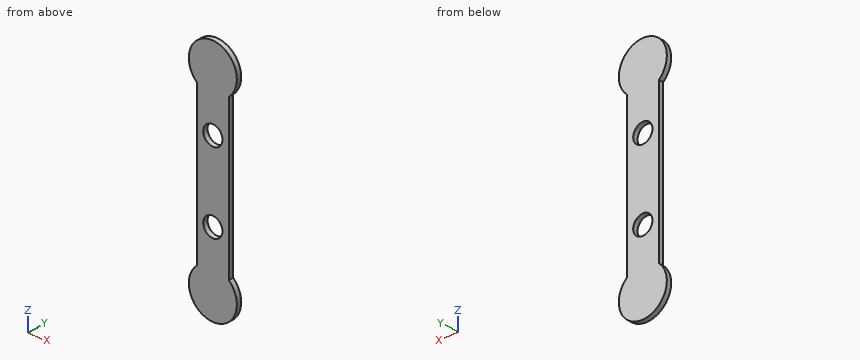
Autodesk Inventor part; units mm, degrees
ref_plane "YZ Plane" through (0, 0, 0) normal (1, 0, 0) x (0, 1, 0)
ref_plane "XZ Plane" through (0, 0, 0) normal (0, 1, 0) x (-1, 0, 0)
ref_plane "XY Plane" through (0, 0, 0) normal (0, 0, 1) x (1, 0, 0)
sketch "Sketch1" plane through (0, 0, 0) normal (0, 1, 0) x (-1, 0, 0)
  line L0 (0, 0) -> (0, 75)
  line L1 (0, 0) -> (0, -75)
  line L2 (0, -75) -> (0, -60)
  circle A0 centre (0, -60) radius 15
  circle A1 centre (0, 60) radius 15
  line L3 (-10, 45) -> (-10, -48.8197)
  line L4 (10, 45) -> (10, -48.8197)
  line L5 (10, 45) -> (10, 48.8197)
  line L6 (-10, 45) -> (-10, 48.8197)
  line L7 (10, 45) -> (-10, 45)
  line L8 (-10, -48.8197) -> (-10, 0)
  line L9 (0, -24.4098) -> (10, -24.4098)
  line L10 (10, 0) -> (0, 0)
  line L11 (0, 24.4098) -> (10, 24.4098)
  line L12 (0, -24.4098) -> (-10, -24.4098)
  line L13 (0, 24.4098) -> (-10, 24.4098)
  circle A2 centre (0, -24.4098) radius 6
  circle A3 centre (0, 24.4098) radius 6
  dimension "d1" = 75
  dimension "d2" = 75
  dimension "d3" = 15
  dimension "d6" = 20
  dimension "d7" = 97.6393
  dimension "d10" = 12
  dimension "d11" = 12
extrude "Extrusion1" add sketch "Sketch1" along normal blind 3 contours L1 A2 L12 L3 L13 A3 L0 | L10 L4 L9 A2 L1 | L0 A3 L11 L4 L10 | L13 L3 L7 L0 A3 | A3 L0 L7 L4 L11 | L9 L4 A0 L1 A2 | A2 L1 A0 L3 L12 | L7 A1 L5 | A0 L1 | A1 L0 | L7 L6 A1 | L0 A1 | L1 A0
properties part number "ramenovaPricka"
Input: part model. Units: mm. Frame: model coordinates. Coordinates: 2 decimals unless noted, no trailing zeros. Loops run counter-clockwise (first coordinate to the right, second up) from the corner with the lowest first, then second, coordinate; pieces in that order, holes last. Notation, with made-up numbers: (-37.75, -21) -> (-15.75, -21) arc R36 cw to (-15.75, 17) -> close; hole circle Ø11 at (89.25, -6). An arc over 180 degrees is marked (long way). Write each question's results on one line, items separated by ' | '. Start each with the question number.
Q1. Pin query (flat end, axial travel): pin 1 (1.5 mm diameter, centred on y = 1, z = 8, fed in from -X); pin 2 (1 mm diameter, centred on x = -12, y = 1, fed in from -Z). Return the tip coordinate at first contact, or that it passes through.
Q2. Section B-B, the plane y = 1.75. Return the cut outline in (x, z).
Q3. Section A-A, the plane x = 0. Return the cut outline in (y, z), plus the area to 3 significant figures.
Q4. Section D-D, the plane z = -43. Return the cut outline in (x, y), plus the area to 3 significant figures.
Q5. Ray query, line 1 (Z direction, x = 0, y = 2.1); line 2 (Z direction, x = 2.75, y = 0.4); line 3 (X direction, y = 2.75, z = 18). Return the intervals inside material, ascending. Write a range as from..to.
Q6. Section C-C, the plane x = -11.25. Return the cut outline in (y, z), plus the area to 3 significant figures.
Found:
1) pin 1: x = -10 | pin 2: z = -69.63
2) outline: (-10, -48.82) arc R15 ccw (long way) to (10, -48.82) -> (10, 48.82) arc R15 ccw (long way) to (-10, 48.82) -> close; hole circle Ø12 at (0, -24.41); hole circle Ø12 at (0, 24.41)
3) outline: (0, -75) -> (3, -75) -> (3, -30.41) -> (0, -30.41) -> close; (0, -18.41) -> (3, -18.41) -> (3, 18.41) -> (0, 18.41) -> close; (0, 30.41) -> (3, 30.41) -> (3, 75) -> (0, 75) -> close | area: 378 mm2
4) outline: (-10, 0) -> (10, 0) -> (10, 3) -> (-10, 3) -> close | area: 60.0 mm2
5) line 1: -75..-30.41, -18.41..18.41, 30.41..75 | line 2: -74.75..-29.74, -19.08..19.08, 29.74..74.75 | line 3: -10..10
6) outline: (0, -69.92) -> (3, -69.92) -> (3, -50.08) -> (0, -50.08) -> close; (0, 50.08) -> (3, 50.08) -> (3, 69.92) -> (0, 69.92) -> close | area: 119 mm2
